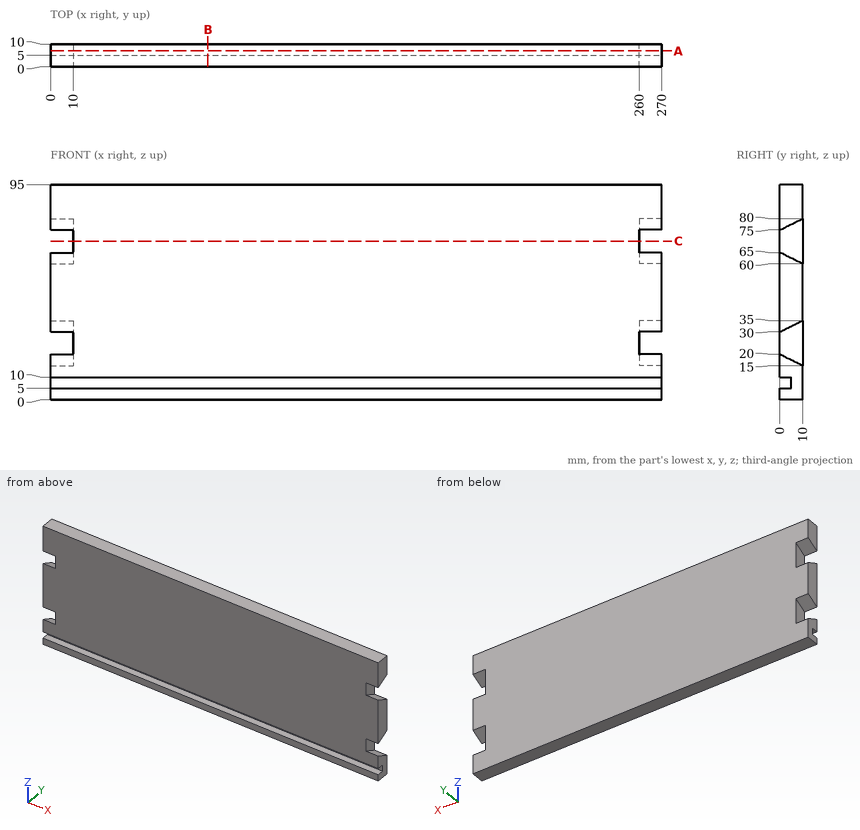
Geometry: see drawing. Coordinates: mm, zero at the bounding-box minimum. Coordinates: 2 decimals unless noted, no trailing zeros. Write each loop counter-clockwise with the first axis right and the second up, starting at its lowest first coordinate (ties: lowest second). Pieces come first, ordered by that corner, then holes. Notation, with made-up numbers: M 21.5,46.5 L 30.5,46.5 A11 ccw 30.5,50.5 Z; hole C 25.25,71 d9. An arc over 180 degrees is marked long. Use CSV: the item, a comma, the result in double quotes. Start each with the question number.
1. First-contact query: P1, Ø5, axis at y = 3, z = 72, coming from the -X side; P2, Ø4, axis at x = 110.5, z = 7.5, coming from the -Y side; P3, Ø3, axis at y = 6, z = 30, coming from the +X side. Flat tips, straight axial feed; report the tip coordinate or a pass-through.
2. Cut plane C-C on z = 70. Return the cut outline in (x, y).
3. Cut plane A-A on y = 7. Return the cut outline in (x, z).
4. Ray query, probe 1 along Z at (x, y) = (165, 2.25); probe 2 along Y at (x, z) = (255, 7.5); probe 3 along X at (y, z) = (9.5, 34). Return the intervals inside material, ascending.
5. Cut plane B-B on x = 69.5. Return the cut outline in (y, z), plus the area to 3 significant figures.
Entries:
1,P1,"x = 10"
1,P2,"y = 5"
1,P3,"x = 260"
2,outline,"M 10,0 L 260,0 L 260,10 L 10,10 Z"
3,outline,"M 0,0 L 270,0 L 270,16.5 L 260,16.5 L 260,33.5 L 270,33.5 L 270,61.5 L 260,61.5 L 260,78.5 L 270,78.5 L 270,95 L 0,95 L 0,78.5 L 10,78.5 L 10,61.5 L 0,61.5 L 0,33.5 L 10,33.5 L 10,16.5 L 0,16.5 Z"
4,probe 1,"0 to 5, 10 to 95"
4,probe 2,"5 to 10"
4,probe 3,"10 to 260"
5,outline,"M 0,0 L 10,0 L 10,95 L 0,95 L 0,10 L 5,10 L 5,5 L 0,5 Z"
5,area,"925 mm²"
